The figure shows three views and two pictorial views of one solid part (mm, origin at its lowest corner). Answer the questions. A direction names the side the tool comes from. Round coordinates to 2 decimals unless told otherwise and drop trailing zeros. Order: outer loops, then holes, each group sorted by start corner. A loop starts at its lowest first (then second) coordinate and runs counter-clockwise, first axis right, second up. Notation, with made-up numbers: (-14.75, -26) - (18.25, -26) arc R23 ccw to (18.25, -8) - close; hole circle Ø3 at (26.25, 62.5). An arc over 180 degrees is marked (long way). One line per item, written item: value. Start each with the question number.
1. A tool of negligible diameter and unlimited length cuts with its end or side. For the marked faces 1 and 2, from which of +Z, -Z, +X, -X, +Y, -Y can it reach the whole face along a straight path? Write none if from no direction.
2. Section A-A, the plane z = 12 is taken. Give the vertices of the cut face in (x, y), then the cut area to 3 significant figures.
3. Section D-D, the plane z = 119.5 is taken. Give the vertices of the cut face in (x, y).
4. A flat-ended cylindrical pin translates along its axis: P1, Ø3, axis at y = 67, z = 108.5, coming from the -X side. Find the tip coordinate at first contact, or state that the pin passes through.
5. Section C-C, the plane x = 54.5 is taken. Give the vertices of the cut face in (y, z), then the cut area to 3 significant figures.
6. Straight lines are drawn through the part: line 1 (Y direction, x = 74, z = 15); line 2 (X direction, y = 50.5, z = 38). For each, find the intervals that lie inside material, in ascending order.
7. Section B-B, the plane y = 65 is taken. Give the vertices of the cut face in (x, z), then the cut area to 3 significant figures.
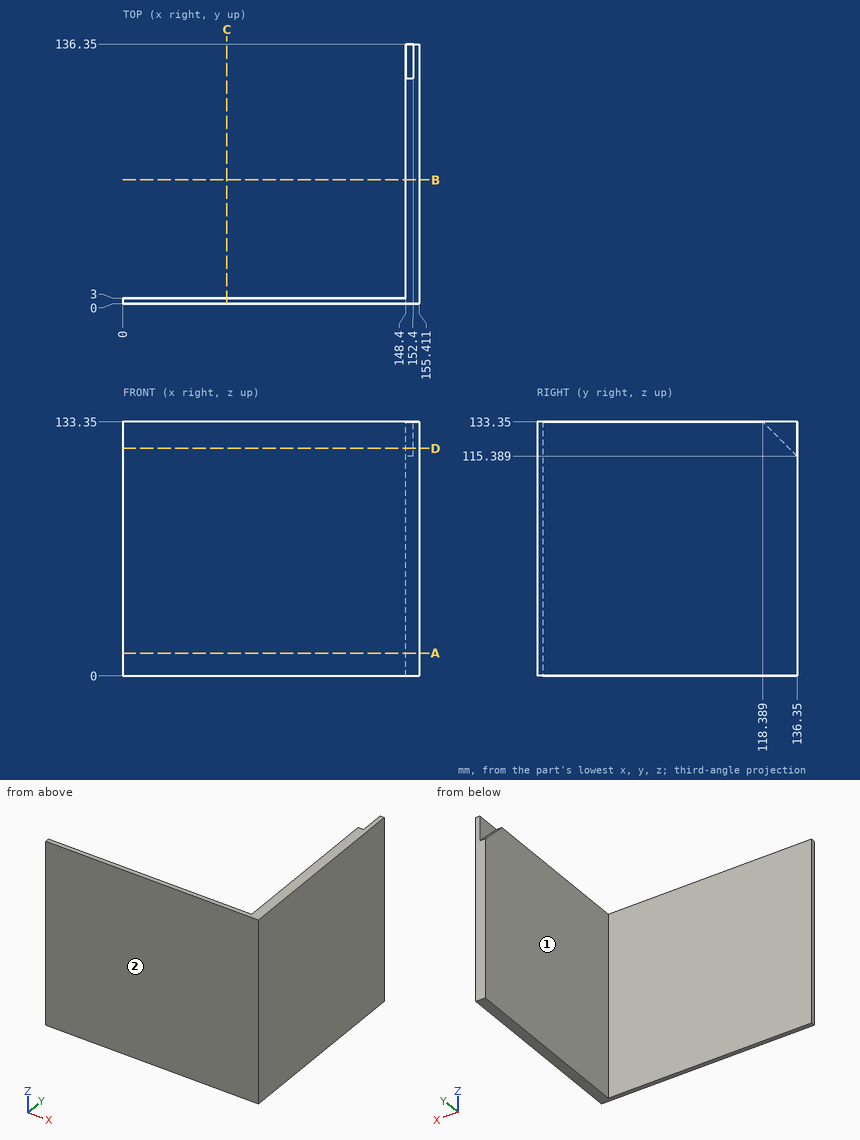
Answer list:
1. face 1: +Z, -Z, -X, +Y
1. face 2: +Z, -Z, +X, -X, -Y
2. outline: (0, 0) - (155.41, 0) - (155.41, 136.35) - (148.4, 136.35) - (148.4, 3) - (0, 3) - close
2. area: 1,400 mm²
3. outline: (0, 0) - (155.41, 0) - (155.41, 136.35) - (152.4, 136.35) - (152.4, 132.24) - (148.4, 132.24) - (148.4, 3) - (0, 3) - close
4. P1: stops at x = 148.4
5. outline: (0, 0) - (3, 0) - (3, 133.35) - (0, 133.35) - close
5. area: 400 mm²
6. line 1: y = 0 to 3
6. line 2: x = 148.4 to 155.41
7. outline: (148.4, 0) - (155.41, 0) - (155.41, 133.35) - (148.4, 133.35) - close
7. area: 935 mm²
